Could you check a few things on this model? Use its own coordinates, in mm. A direction names the side the tool comes from. Give positions to 0.01 mm unless a question says otherwise; leave off trailing zeros. Loops run counter-clockwise (first coordinate to the right, second up) from the corner with the lowest first, then second, coordinate; pieces in that order, holes last. Notation, with made-up numbers: M 48,54.5 L 84,54.5 A15 cw 84,62.5 Z; hole C 73,43.5 d3. An arc over 180 degrees is marked long. Answer in a Markdown table with one row per item. Add a question column.
1. If we section it at C-C on x = 24: List the corners of the cut face in (y, z) for me.
2. I need wall thicknesses on line 1 along Y through (x, z) = (11, 6); line 2 along X through (y, z) = (36, 6); line 3 along X through (y, z) = (41.5, 4.5). Which ranges of each line are inside material? Lowest first, please. Write a range as from..to.
3. Which directions (+Z, -Z, +X, -X, +Y, -Y) give clear straight access to the entire face, cutting with the end or side of a thin tool? Please do faces 1 (the flat face through (8.018, 39, 4)), 2 (the flat face through (52.412, 29, 3)).
4. If we section it at A-A on z = 3.5: List the corners of the cut face in (x, y) for me.
5. I'm going to push flat-ended pins straight in: pin 1 Ø15 at (x, y) = (38.5, 33.5) entering from +Z; pin 2 Ø0.6 at (x, z) = (7, 3) entering from -Y. Where does each tip first touch, or does it pass through?
6. Thinking about a two-plate mould opening in Y: for faces 3 (the flat face through (26, 29, 0)), 4 (the flat face through (26, 0, 3)), 5 (the flat face through (26, 56.831, 4)), which applies, released by +Y, released by -Y, zero draft, split by the parting line, or undercut?
7. If we section it at B-B on y = 4: List the corners of the cut face in (x, z) for me.
8. If we section it at D-D on y = 47: List the corners of the cut face in (x, z) for me.
```python
from build123d import *

# Parameters (mm, degrees)
F0_W     = 52.411996
F0_H     = 58.101058
F1_DEPTH = 6.35
F2_T     = -1.27
F3_W     = 1.273277
F3_H     = 38.1
F4_DEPTH = 6.35
F5_W     = 5.08
F5_H     = 1.27
F6_DEPTH = 6.35


with BuildPart() as f1:
    # F0 (on Top) → F1 (new body)
    with BuildSketch(Plane.XY):
        with Locations((26.205998, 29.050529)):
            Rectangle(F0_W, F0_H)
    extrude(amount=F1_DEPTH)

    # F2
    f2_openings = [f1.faces().sort_by_distance(p)[0] for p in [
        (26.205998, 29.050529, 6.35),
    ]]
    offset(amount=F2_T, openings=f2_openings)

    # F3 (on Top) → F4 (join)
    with BuildSketch(Plane.XY):
        with Locations((6.968005, 20.351489)):
            Rectangle(F3_W, F3_H)
    extrude(amount=F4_DEPTH)

    # F5 (on Top) → F6 (join)
    with BuildSketch(Plane.XY):
        with Locations((10.558338, 38.800815)):
            Rectangle(F5_W, F5_H)
    extrude(amount=F6_DEPTH)


solid = f1.part
```
Results:
| question | item | result |
|---|---|---|
| 1 | outline | M 0,0 L 58.1,0 L 58.1,6.35 L 56.83,6.35 L 56.83,1.27 L 1.27,1.27 L 1.27,6.35 L 0,6.35 Z |
| 2 | line 1 | 0..1.27, 38.17..39.44, 56.83..58.1 |
| 2 | line 2 | 0..1.27, 6.33..7.6, 51.14..52.41 |
| 2 | line 3 | 0..1.27, 51.14..52.41 |
| 3 | face 1 | +Z |
| 3 | face 2 | +Z, -Z, +X, +Y, -Y |
| 4 | outline | M 0,0 L 52.41,0 L 52.41,58.1 L 0,58.1 Z; M 6.33,1.3 L 7.6,1.3 L 7.6,39.4 L 6.33,39.4 Z; M 8.02,38.17 L 13.1,38.17 L 13.1,39.44 L 8.02,39.44 Z; hole M 1.27,1.27 L 51.14,1.27 L 51.14,56.83 L 1.27,56.83 Z |
| 5 | pin 1 | z = 1.27 |
| 5 | pin 2 | y = 0 |
| 6 | face 3 | zero draft |
| 6 | face 4 | released by -Y |
| 6 | face 5 | undercut |
| 7 | outline | M 0,0 L 52.41,0 L 52.41,6.35 L 51.14,6.35 L 51.14,1.27 L 7.6,1.27 L 7.6,6.35 L 6.33,6.35 L 6.33,1.27 L 1.27,1.27 L 1.27,6.35 L 0,6.35 Z |
| 8 | outline | M 0,0 L 52.41,0 L 52.41,6.35 L 51.14,6.35 L 51.14,1.27 L 1.27,1.27 L 1.27,6.35 L 0,6.35 Z |
